Source: CAD feature listing. Evaluate the final solid. Frame: model axes, mm. Face numbers are marked on the shaded views. A direction names the side the tool comes from. Coordinates: 2 decimals unless noted, no trailing zeros. Write each loop counter-clockwise with the first axis right and the second up, starting at its lowest first coordinate (ties: lowest second). Pieces come first, ordered by that corner, then holes. Notation, with made-up numbers: M 54.5,23.5 L 111.5,23.5 A18 cw 111.5,48.5 Z; hole C 35,13.5 d1. An arc over 180 degrees is marked long. One line per item, written item: value. Start each with the question number.
Item 1: Set-up query: the marked faces 4, 5 and 6. Return all of +Z, -Z, +X, -X, +Y, -Y with unobstructed straight access to the full face (end or side cutting, diameter ignored); none if empty.
Item 2: Mould query, pull axis X, two halves, no side actions, for the marked faces 1, 2 and 3. Classes: released by +X, released by -X, zero draft, split by the parting line, or undercut.
Item 3: Cut plane A-A, the plane y = -4.5. Output: boundary loops of the cut face in (x, z), then the cut area to 3 significant figures.
Item 4: Cut plane C-C, the plane y = -0.25. Output: boundary loops of the cut face in (x, z).
Item 5: Cut plane D-D, the plane z = 4.5. Output: boundary loops of the cut face in (x, y), then the cut area to 3 significant figures.
Item 6: Cut plane B-B, the plane x = 5.5. Output: boundary loops of the cut face in (y, z), then the cut area to 4 significant figures.
Item 7: Pin query (flat end, axial travel): P1, Ø1.8, axis at x = 1.5, y = 5.5, coming from the +Z side; P2, Ø0.8, axis at x = -4.5, z = 2.5, coming from the -Y side; P3, Ø1.8, axis at x = -7.5, y = 4.5, coming from the +Z side; P4, Ø1.8, axis at x = 1.5, y = 2, coming from the +Z side. Return the tip coordinate at first contact, or that it passes through.
Item 8: Ray query, L1, parallel to Y at x = -7.5, z = 1.9; L2, parallel to X at y = -5, z = 5; L3, parallel to X at y = -1.25, z = 6.75. Return the intervals inside material, ascending. Write a range as from..to.
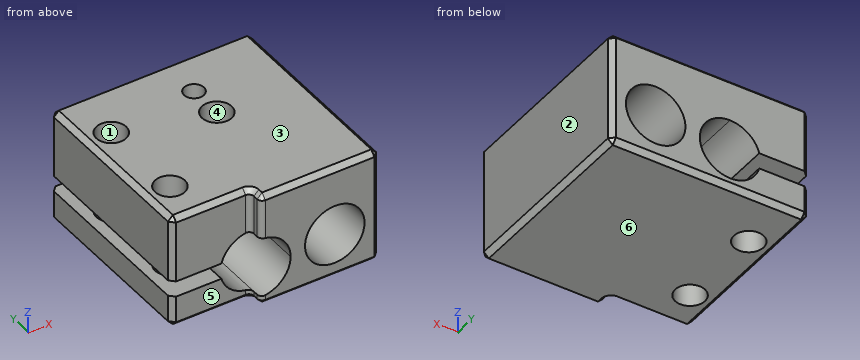
```python
from build123d import *

# Parameters (mm, degrees)
BOSS_EXTRUDE1_DEPTH = 11.5
SKETCH2_R           = 1.5
CUT_EXTRUDE1_DEPTH  = 12.5
SKETCH2_3_R         = 0.75
CUT_EXTRUDE2_DEPTH  = 4.5
SKETCH2_4_R         = 1
CUT_EXTRUDE3_DEPTH  = 2
SKETCH2_5_R         = 1.5
CUT_EXTRUDE4_DEPTH  = 3.5
CUT_EXTRUDE5_DEPTH  = 21
SKETCH3_4_R         = 3
CUT_EXTRUDE6_DEPTH  = 21
FILLET1_R           = 0.5
CHAMFER1_SIZE       = 0.5


with BuildPart() as part:
    # Sketch1 → Boss-Extrude1 (new body)
    with BuildSketch(Plane.XY):
        Polygon((-10, 10), (10, 10), (10, -10), (-2, -10), (-2, -8.5), (-10, -8.5), align=None)
    extrude(amount=BOSS_EXTRUDE1_DEPTH)

    # Sketch2 → Cut-Extrude1 (cut, through all)
    with BuildSketch(Plane.XY.offset(11.5)):
        with Locations((-7.5, 4.5)):
            Circle(SKETCH2_R)
        with Locations((-7.5, -4.5)):
            Circle(SKETCH2_R)
    extrude(amount=-CUT_EXTRUDE1_DEPTH, mode=Mode.SUBTRACT)

    # Sketch2_3 → Cut-Extrude2 (cut)
    with BuildSketch(Plane.XY.offset(11.5)):
        with Locations((1.5, 5.5)):
            Circle(SKETCH2_3_R)
    extrude(amount=-CUT_EXTRUDE2_DEPTH, mode=Mode.SUBTRACT)

    # Sketch2_4 → Cut-Extrude3 (cut)
    with BuildSketch(Plane.XY.offset(11.5)):
        with Locations((1.5, 5.5)):
            Circle(SKETCH2_4_R)
    extrude(amount=-CUT_EXTRUDE3_DEPTH, mode=Mode.SUBTRACT)

    # Sketch2_5 → Cut-Extrude4 (cut)
    with BuildSketch(Plane.XY.offset(11.5)):
        with Locations((1.5, 2)):
            Circle(SKETCH2_5_R)
    extrude(amount=-CUT_EXTRUDE4_DEPTH, mode=Mode.SUBTRACT)

    # Sketch3 → Cut-Extrude5 (cut, through all)
    with BuildSketch(Plane.XZ.offset(10)):
        with BuildLine():
            Line((-4.943212531, 4.8), (-10, 4.8))
            Line((-10, 4.8), (-10, 3.2))
            Line((-10, 3.2), (-4.943212531, 3.2))
            ThreePointArc((-4.943212531, 3.2), (-5.05, 4), (-4.943212531, 4.8))
        make_face()
        with BuildLine():
            ThreePointArc((-2, 7.05), (-3.852363355, 6.423066239), (-4.943212531, 4.8))
            ThreePointArc((-4.943212531, 4.8), (-5.05, 4), (-4.943212531, 3.2))
            ThreePointArc((-4.943212531, 3.2), (-3.852363355, 1.576933761), (-2, 0.95))
            Line((-2, 0.95), (-2, 7.05))
        make_face()
        with BuildLine():
            ThreePointArc((1.05, 4), (0.156675683, 6.156675683), (-2, 7.05))
            Line((-2, 7.05), (-2, 0.95))
            ThreePointArc((-2, 0.95), (0.156675683, 1.843324317), (1.05, 4))
        make_face()
    extrude(amount=-CUT_EXTRUDE5_DEPTH, mode=Mode.SUBTRACT)

    # Sketch3_4 → Cut-Extrude6 (cut, through all)
    with BuildSketch(Plane.XZ.offset(10)):
        with Locations((5.5, 4.5)):
            Circle(SKETCH3_4_R)
    extrude(amount=-CUT_EXTRUDE6_DEPTH, mode=Mode.SUBTRACT)

    # Fillet1
    fillet1_edges = [part.edges().sort_by_distance(p)[0] for p in [
        (-2, -10, 9.275),
        (-2, -8.5, 9.275),
        (-2, -10, 0.475),
        (-2, -8.5, 0.475),
    ]]
    fillet(fillet1_edges, radius=FILLET1_R)

    # Chamfer1
    chamfer1_edges = [part.edges().sort_by_distance(p)[0] for p in [
        (-10, 0.75, 11.5),
        (10, -10, 5.75),
        (-10, -8.5, 8.15),
        (-10, 10, 8.15),
        (10, 10, 5.75),
        (-6.25, -8.5, 11.5),
        (10, 0, 11.5),
        (-10, -8.5, 1.6),
        (-10, 10, 1.6),
        (-6.25, -8.5, 0),
        (0, 10, 11.5),
        (-10, 0.75, 0),
        (0, 10, 0),
        (-2, -9.25, 0),
        (10, 0, 0),
        (4.25, -10, 0),
        (4.25, -10, 11.5),
        (-2, -9.25, 11.5),
        (-1.853553391, -9.853553391, 11.5),
        (-1.853553391, -9.853553391, 0),
        (-2.146446609, -8.646446609, 0),
        (-2.146446609, -8.646446609, 11.5),
    ]]
    chamfer(chamfer1_edges, length=CHAMFER1_SIZE)


solid = part.part
```
From the geometry:
1. face 4: +Z
1. face 5: +Z, -Z, -X, -Y
1. face 6: -Z, +X, -X, +Y, -Y
2. face 1: undercut
2. face 2: released by +X
2. face 3: zero draft
3. outline: M -10,0.5 L -9.5,0 L -9,0 L -9,3.2 L -10,3.2 Z; M -10,4.8 L -9,4.8 L -9,11.5 L -9.5,11.5 L -10,11 Z; M -6,0 L 9.5,0 L 10,0.5 L 10,11 L 9.5,11.5 L -6,11.5 L -6,4.8 L -4.94,4.8 A3.05 cw long -4.94,3.2 L -6,3.2 Z; hole C 5.5,4.5 d6
3. area: 134 mm²
4. outline: M -10,0.5 L -9.5,0 L 9.5,0 L 10,0.5 L 10,11 L 9.5,11.5 L -9.5,11.5 L -10,11 L -10,4.8 L -4.94,4.8 A3.05 cw long -4.94,3.2 L -10,3.2 Z; hole C 5.5,4.5 d6
5. outline: M 1.01,-10 L 2.5,-10 L 2.5,10 L 1.01,10 Z; M 8.5,-10 L 9.5,-10 L 10,-9.5 L 10,9.5 L 9.5,10 L 8.5,10 Z
5. area: 59.6 mm²
6. outline: M -10,0.5 L -9.5,0 L 9.5,0 L 10,0.5 L 10,1.5 L -10,1.5 Z; M -10,7.5 L 10,7.5 L 10,11 L 9.5,11.5 L -9.5,11.5 L -10,11 Z
6. area: 109.5 mm²
7. P1: stops at z = 9.5
7. P2: stops at y = -8.5
7. P3: passes through
7. P4: stops at z = 8
8. L1: y = -8.5..-6, -3..3, 6..10
8. L2: x = -10..-8.91, -6.09..-4.88, 0.88..2.54, 8.46..10
8. L3: x = -10..-3.32, -0.68..3.52, 7.48..10
